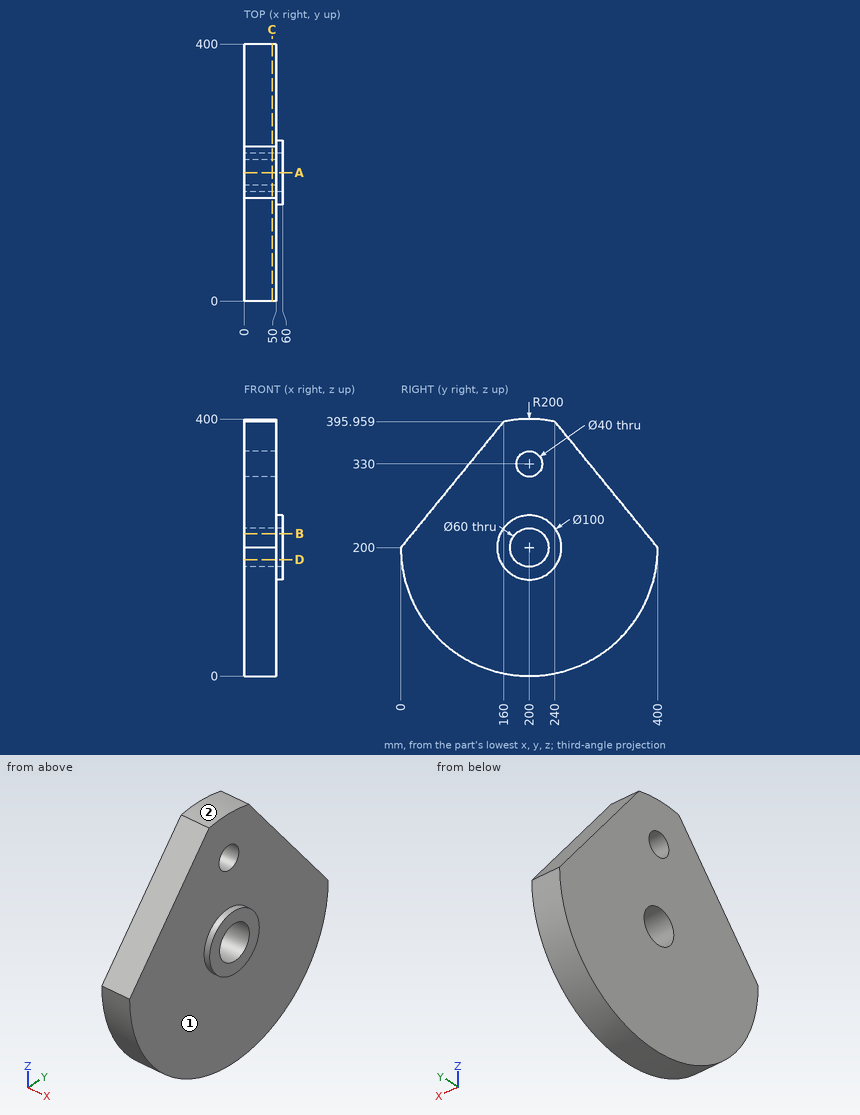
Input: dimensioned drawing with shaded views. Units: mm. Origin: part minimum x, y, z. A direction names the side the tool comes from. Coordinates: 2 decimals unless noted, no trailing zeros. Loops run counter-clockwise (first coordinate to the right, second up) from the corner with the lowest first, then second, coordinate; pieces in that order, holes last. Notation, with made-up numbers: M -21,24.25 L 6,24.25 A30 ccw 6,54.25 Z; hole C 88.5,-32 d6. An arc over 180 degrees is marked long. Use a Markdown table: item, result. Add a question column.
Q1. First-contact query: pin 1 (12 mm diameter, centred on x = 41.5, z = 158, fed in from -Y); pin 2 (1.5 mm diameter, centred on x = 13, y = 145.5, fed in from -Z); pin 3 (3 mm diameter, centred on x = 29.5, y = 104.5, fed in from -Z). Flat tips, straight axial feed; report the tip coordinate or a pass-through.
Q2. Section query C-C, the plane x = 43.5. Return loops of the section in (y, z).
Q3. Section query A-A, the plane y = 200. Return loops of the section in (x, z).
Q4. Access query for the marked faces 1 and 2. Directions: +Z, -Z, +X, -X, +Y, -Y. A direction counts if a zero-diameter tool reaches every point of the face in a straight line with its end or side. Return the directions, or none.
Q5. Section query B-B, the plane z = 221.5. Return loops of the section in (x, y) (1 decimal), and give its area (3 significant figures).
Q6. Material intervals for L1, parallel to Z at x = 21.5, y = 200; L2, parallel to X at y = 257.5, z = 130.5; L3, parallel to Y at x = 49.5, z = 341, sorted ascending.
Q7. Section query D-D, the plane z = 181. Return loops of the section in (x, y).
Result:
| question | item | result |
|---|---|---|
| 1 | pin 1 | stops at y = 3.27 |
| 1 | pin 2 | stops at z = 7.36 |
| 1 | pin 3 | stops at z = 23.47 |
| 2 | outline | M 0,200 A200 ccw 400,200 L 240,395.96 A200 ccw 160,395.96 Z; hole C 200,200 d60; hole C 200,330 d40 |
| 3 | outline | M 0,0 L 50,0 L 50,150 L 60,150 L 60,170 L 0,170 Z; M 0,230 L 60,230 L 60,250 L 50,250 L 50,310 L 0,310 Z; M 0,350 L 50,350 L 50,400 L 0,400 Z |
| 4 | face 1 | +X |
| 4 | face 2 | +Z, +X, -X |
| 5 | outline | M 0,17.6 L 50,17.6 L 50,154.9 L 60,154.9 L 60,179.1 L 0,179.1 Z; M 0,220.9 L 60,220.9 L 60,245.1 L 50,245.1 L 50,382.4 L 0,382.4 Z |
| 5 | area | 16,600 mm2 |
| 6 | L1 | z = 0 to 170, 230 to 310, 350 to 400 |
| 6 | L2 | x = 0 to 50 |
| 6 | L3 | y = 115.13 to 183.3, 216.7 to 284.87 |
| 7 | outline | M 0,0.9 L 50,0.9 L 50,153.75 L 60,153.75 L 60,176.78 L 0,176.78 Z; M 0,223.22 L 60,223.22 L 60,246.25 L 50,246.25 L 50,399.1 L 0,399.1 Z |
